Geometry check sheet. Reference: the model listing, model coordinates, mm. A direction names the side the tool comes from. Round coordinates to 2 decimals unless told otherwise and drop trailing zeros. Order: outer loops, then holes, each group sorted by start corner. A loop starts at its lowest first (then second) coordinate and runs counter-clockwise, first axis right, second up.
(1) Release check for a two-part mould opening along Z. For faces 1 (the face through (-15, 34, 25)), 2 (the face through (3.226, 47, 0)), 3 (the face through (-64.294, 5, 0)) record: +Z half, -Z half, draft (parallel to the pull), parting line (faces both ways), or undercut.
(2) Sectioned sample at C-C (y = 63). Record the boundary of the cut face in (x, z).
(3) Sectioned sample at B-B (x = -42.5). Record the boundary of the cut face in (y, z), plus the area to 3 significant figures.
(4) Sectioned sample at A-A (z = 5). Record the boundary of the cut face in (x, y).
(5) Go/stop test with flat-tipped pins: pin 1 (20 mm diameter, centred on x = 13.5, z = 6, fed in from +Y); pin 2 (2 mm diameter, centred on x = 21, z = 3.5, fed in from +Y); pin 3 (3 mm diameter, centred on x = -36.5, z = 12.5, fed in from +Y). Record where each tip stops, or that it passes through.
(6) Set-up check for faces 4 (the face through (-41, 24.458, 0)), 5 (the face through (-40.774, 55, 20)), 6 (the face through (9.226, 55, 20)), 7 (the face through (-16, 77.458, 0)): record each of +Z, -Z, +X, -X, +Y, -Y from which the full face is reachable in a straight line by a thin tool's end or side.
(7) Sectioned sample at D-D (z = -20). Record the boundary of the cut face in (x, y).
(8) Material ranges on line 1 along Z through (x, y) = (-34.5, 60.5); line 2 along X through (y, z) = (54, 3.5); line 3 along X through (y, z) = (31, -7), recorded low to high.
from build123d import *

# Parameters (mm, degrees)
BOSS_EXTRUDE1_DEPTH = 25
SKETCH3_W           = 6
SKETCH3_H           = 30
SKETCH3_W_2         = 12
CUT_EXTRUDE2_DEPTH  = 45
SKETCH4_W           = 41.759295091
SKETCH4_H           = 20
CUT_EXTRUDE4_DEPTH  = 7


with BuildPart() as part:
    # Sketch1 → Boss-Extrude1 (new, symmetric)
    with BuildSketch(Plane.XY):
        with BuildLine():
            Line((9.225854521, 69.458085549), (-0.764451304, 69.458085549))
            ThreePointArc((-0.764451304, 69.458085549), (-15.754659065, 85), (-30.744866826, 69.458085549))
            Line((-30.744866826, 69.458085549), (-40.774145479, 69.458085549))
            Line((-40.774145479, 69.458085549), (-40.774145479, 40))
            Line((-40.774145479, 40), (-45.774145479, 40))
            Line((-45.774145479, 40), (-64.293941681, 10))
            Line((-64.293941681, 10), (-64.293941681, 0))
            Line((-64.293941681, 0), (-35.754659065, 0))
            ThreePointArc((-35.754659065, 0), (-15.754659065, 20), (4.245340935, 0))
            Line((4.245340935, 0), (35.706058319, 0))
            Line((35.706058319, 0), (35.706058319, 10))
            Line((35.706058319, 10), (14.225854521, 40))
            Line((14.225854521, 40), (9.225854521, 40))
            Line((9.225854521, 40), (9.225854521, 69.458085549))
        make_face()
    extrude(amount=BOSS_EXTRUDE1_DEPTH, both=True)

    # Sketch3 → Cut-Extrude2 (cut)
    with BuildSketch(Plane(origin=(0, 69.458085549, 0), x_dir=(1, 0, 0), z_dir=(0, 1, 0))):
        with Locations((6.225854521, 0)):
            Rectangle(SKETCH3_W, SKETCH3_H)
        with Locations((15.225854521, 0)):
            Rectangle(SKETCH3_W_2, SKETCH3_H)
    cut_extrude2 = extrude(amount=-CUT_EXTRUDE2_DEPTH, mode=Mode.SUBTRACT)

    # Mirror1: Cut-Extrude2 across plane
    add(cut_extrude2.mirror(Plane.ZY.offset(14.293941681)), mode=Mode.SUBTRACT)

    # Sketch4 → Cut-Extrude4 (cut, symmetric)
    with BuildSketch(Plane(origin=(0, 84.458085549, 0), x_dir=(1, 0, 0), z_dir=(0, 1, 0))):
        with Locations((-15.754659066, 0)):
            Rectangle(SKETCH4_W, SKETCH4_H)
    extrude(amount=CUT_EXTRUDE4_DEPTH, both=True, mode=Mode.SUBTRACT)


solid = part.part
Answer below:
1. face 1: +Z half
1. face 2: undercut
1. face 3: draft
2. outline: (-40.77, -25) - (9.23, -25) - (9.23, -15) - (3.23, -15) - (3.23, 15) - (9.23, 15) - (9.23, 25) - (-40.77, 25) - (-40.77, 15) - (-31.81, 15) - (-31.81, -15) - (-40.77, -15) - close
3. outline: (0, -25) - (40, -25) - (40, -15) - (24.46, -15) - (24.46, 15) - (40, 15) - (40, 25) - (0, 25) - close
3. area: 1,530 mm2
4. outline: (-64.29, 0) - (-35.75, 0) arc R20 cw to (4.25, 0) - (35.71, 0) - (35.71, 10) - (21.23, 30.22) - (21.23, 24.46) - (3.23, 24.46) - (3.23, 69.46) - (-0.76, 69.46) arc R15 ccw to (-2.74, 77.46) - (-28.77, 77.46) arc R15 ccw to (-30.74, 69.46) - (-31.81, 69.46) - (-31.81, 24.46) - (-49.81, 24.46) - (-49.81, 33.46) - (-64.29, 10) - close
5. pin 1: stops at y = 69.46
5. pin 2: stops at y = 30.22
5. pin 3: stops at y = 24.46
6. face 4: +Y
6. face 5: +Z, -Z, -X, +Y
6. face 6: +Z, -Z, +X, +Y
6. face 7: +X, -X, +Y
7. outline: (-64.29, 0) - (-35.75, 0) arc R20 cw to (4.25, 0) - (35.71, 0) - (35.71, 10) - (14.23, 40) - (9.23, 40) - (9.23, 69.46) - (-0.76, 69.46) arc R15 ccw (long way) to (-30.74, 69.46) - (-40.77, 69.46) - (-40.77, 40) - (-45.77, 40) - (-64.29, 10) - close
8. line 1: z = -25 to -15, 15 to 25
8. line 2: x = -31.81 to 3.23
8. line 3: x = -51.33 to -49.81, -31.81 to 3.23
